Can you work these out from the model? Positions are in its coordinate system, mm. A direction names the side the tool comes from. Give positions to 0.01 mm unless a question says otherwise; leave off trailing zeros. Loops run counter-clockwise (first coordinate to the right, second up) from the corner with the lowest first, then second, coordinate; pieces in that order, holes last. Notation, with made-up numbers: (17, 19) - (67, 19) arc R7 ccw to (67, 26) - close; hole circle Ø8 at (13.25, 50). An arc over 180 degrees is marked (long way). Answer as a JSON object with one key per item and string values.
Autodesk Inventor part; units mm, degrees
ref_plane "YZ Plane" through (0, 0, 0) normal (1, 0, 0) x (0, 1, 0)
ref_plane "XZ Plane" through (0, 0, 0) normal (0, 1, 0) x (-1, 0, 0)
ref_plane "XY Plane" through (0, 0, 0) normal (0, 0, 1) x (1, 0, 0)
sketch "Sketch1" plane through (0, 0, 0) normal (0, 0, 1) x (1, 0, 0)
  circle A0 centre (0, 0) radius 8
  circle A1 centre (0, -25) radius 8
  line L0 (0, 0) -> (0, -25) construction
  line L1 (-18, 17.5) -> (18, 17.5)
  line L2 (18, 17.5) -> (18, -42.5)
  line L3 (18, -42.5) -> (-18, -42.5)
  line L4 (-18, -42.5) -> (-18, 17.5)
  line L5 (-18, 17.5) -> (18, -42.5) construction
  line L6 (18, 17.5) -> (-18, -42.5) construction
  line L7 (-6, 17.5) -> (6, 17.5)
  line L8 (6, 17.5) -> (6, 11.5)
  line L9 (6, 11.5) -> (-6, 11.5)
  line L10 (-6, 11.5) -> (-6, 17.5)
  line L11 (-6, -42.5) -> (6, -42.5)
  line L12 (6, -42.5) -> (6, -36.5)
  line L13 (6, -36.5) -> (-6, -36.5)
  line L14 (-6, -36.5) -> (-6, -42.5)
  line L15 (-18, -31) -> (-12, -31)
  line L16 (-12, -31) -> (-12, -19)
  line L17 (-12, -19) -> (-18, -19)
  line L18 (-18, -19) -> (-18, -31)
  line L19 (-18, -6) -> (-12, -6)
  line L20 (-12, -6) -> (-12, 6)
  line L21 (-12, 6) -> (-18, 6)
  line L22 (-18, 6) -> (-18, -6)
  line L23 (18, -6) -> (12, -6)
  line L24 (12, -6) -> (12, 6)
  line L25 (12, 6) -> (18, 6)
  line L26 (18, 6) -> (18, -6)
  line L27 (18, -31) -> (12, -31)
  line L28 (12, -31) -> (12, -19)
  line L29 (12, -19) -> (18, -19)
  line L30 (18, -19) -> (18, -31)
  point P0 (0, -12.5)
  point P1 (0, 11.5)
  point P2 (0, 17.5)
  point P3 (12, 0)
  point P4 (-12, 0)
  point P5 (-12, -25)
  point P6 (12, -25)
  dimension "d0" = 16
  dimension "d1" = 25
  dimension "d2" = 36
  dimension "d3" = 60
  dimension "d4" = 12
  dimension "d5" = 6
extrude "Plate1" add sketch "Sketch1" along normal blind 6 contours A0 | A1 | L1 L10 L9 L8 L2 L25 L24 L23 L29 L28 L27 L3 L12 L13 L14 L4 L15 L16 L17 L19 L20 L21
equation "\"d7\" = Thickness"
equation "\"BendRadius\" = Thickness"
equation "\"BendReliefWidth\" = Thickness"
equation "\"BendReliefDepth\" = 0.5 * Thickness"
equation "\"CornerReliefSize\" = 4 * Thickness"
equation "\"MinimumRemnant\" = 2 * Thickness"
equation "\"TransitionRadius\" = BendRadius"
equation "\"JacobiRadiusSize\" = BendRadius"
equation "\"GapSize\" = Thickness"
properties part number "achterkant knoppendoosje" material "Wood (Birch)"
1) Which directions (+Z, -Z, +X, -X, +Y, -Y) give clear straight access to the entire face, cutting with the end or side of a thin tool? Please do faces 1 (the flat face through (-15, -31, 3)), 2 (the flat face through (0, -12, 0)), 3 (the flat face through (6, 15, 3)), 4 (the flat face through (-12, -42.5, 3)), 5 (the flat face through (15, -19, 3)).
Check sheet entries:
{"face 1": "+Z, -Z, -X", "face 2": "-Z, +X, -X, +Y, -Y", "face 3": "+Z, -Z, +Y", "face 4": "+Z, -Z, +X, -X, -Y", "face 5": "+Z, -Z, +X"}
2) Imagine slicing it at D-D on y = -25. Write out the boundary of the cut face in (x, z), and give its area (3 significant figures).
Check sheet entries:
{"outline": "(-12, 0) - (12, 0) - (12, 6) - (-12, 6) - close", "area": "144 mm2"}
3) I need wall thicknesses on L1, parallel to Y at x = 14, z = 2.2; L2, parallel to X at y = 12.5, z = 2.3; L3, parallel to X at y = 3.5, z = 0.8. Which ranges of each line are inside material? Lowest first, please.
Check sheet entries:
{"L1": "-42.5 to -31, -19 to -6, 6 to 17.5", "L2": "-18 to -6, 6 to 18", "L3": "-12 to 12"}
4) Imagine slicing it at C-C on z = 1.7. Write out the boundary of the cut face in (x, y).
Check sheet entries:
{"outline": "(-18, -42.5) - (-6, -42.5) - (-6, -36.5) - (6, -36.5) - (6, -42.5) - (18, -42.5) - (18, -31) - (12, -31) - (12, -19) - (18, -19) - (18, -6) - (12, -6) - (12, 6) - (18, 6) - (18, 17.5) - (6, 17.5) - (6, 11.5) - (-6, 11.5) - (-6, 17.5) - (-18, 17.5) - (-18, 6) - (-12, 6) - (-12, -6) - (-18, -6) - (-18, -19) - (-12, -19) - (-12, -31) - (-18, -31) - close"}
5) If we mould it in two halves opening along X, with no side actions, what happens to faces 6 (the flat face through (-6, -39, 3)), 7 (the flat face through (0, 11.5, 3)), 8 (the flat face through (12, 0, 3)), 9 (the flat face through (-15, -19, 3))? For each: released by +X, released by -X, zero draft, split by the parting line, or undercut.
Check sheet entries:
{"face 6": "undercut", "face 7": "undercut", "face 8": "released by +X", "face 9": "zero draft"}
6) Imagine slicing it at A-A on x = 13. Write out the boundary of the cut face in (y, z).
Check sheet entries:
{"outline": "(-42.5, 0) - (-31, 0) - (-31, 6) - (-42.5, 6) - close; (-19, 0) - (-6, 0) - (-6, 6) - (-19, 6) - close; (6, 0) - (17.5, 0) - (17.5, 6) - (6, 6) - close"}
7) I'm going to push flat-ended pins straight in: P1, Ø1.8, axis at x = -2.5, z = 3.5, coming from the +Y side; P2, Ø1.8, axis at y = -23, z = 3, coming from the -X side; P3, Ø3, axis at x = -3, z = 3, coming from the -Y side. Where does each tip first touch, or does it pass through?
Check sheet entries:
{"P1": "y = 11.5", "P2": "x = -12", "P3": "y = -36.5"}
8) Imagine slicing it at B-B on y = -37.5. Write out the boundary of the cut face in (x, z), and give its area (3 significant figures).
Check sheet entries:
{"outline": "(-18, 0) - (-6, 0) - (-6, 6) - (-18, 6) - close; (6, 0) - (18, 0) - (18, 6) - (6, 6) - close", "area": "144 mm2"}
